Here's how the part is built. I have some questions about the finished solid (model axes, mm). A direction names the side the tool comes from. Round coordinates to 2 decimals unless told otherwise and drop trailing zeros. Write each loop counter-clockwise with the first axis right and the second up, starting at its lowest first coordinate (ties: lowest second). Pieces come first, ordered by that corner, then holes. Notation, with made-up numbers: M 53,1 L 88,1 A19 cw 88,23 Z; hole C -0.5,9.25 d9. An arc over 180 degrees is marked long. Write item = value, one per line. Start each with the question number.
(1) Will these pins go through, and if not, where does the flat tip stop? pin 1 Ø7 at (x, z) = (8, -20) entering from +Y; pin 2 Ø1.6 at (x, z) = (-12.5, -1) entering from -Y; pin 3 Ø3 at (x, y) = (19, 14) entering from -Z; pin 4 Ø8 at (y, z) = (7.5, -13.5) entering from -X.
(2) I want a section at A-A (x = 19.85). List the corners of the cut face in (y, z) for me, and give its area (3 significant figures).
(3) I want a section at C-C (x = 7.05). List the corners of the cut face in (y, z) for me.
(4) I need wall thicknesses on line 1 along X through (y, z) = (21, -1); line 2 along X through (y, z) = (1.05, -41.8); line 3 along Z through (x, y) = (-7.5, 13). Which ranges of each line are inside material? Lowest first, please.
(5) On a 3-axis mill with a long thin cutter (end or side, diameter ignored), from which of +Z, -Z, +X, -X, +Y, -Y can I reach the whole of each face in a straight line? I mean faces 5 (the flat face through (7, 18, -2)), 6 (the flat face through (14.1, 1.6, -19.5)), 7 (the flat face through (32.05, 21, -1)), 8 (the flat face through (-9, 10, -1)), 9 (the cylindrical face through (12.45, 13.45, -0.99)). Say none if no direction works.
(6) I want a section at B-B (y = 21.5). List the corners of the cut face in (x, z) for me, and give its area (3 significant figures).
(7) I want a section at D-D (z = -40.5). List the corners of the cut face in (x, y) for me, and give its area (3 significant figures).
(8) If we mould it in two halves opening along Y, with no side actions, what happens to faces 1 (the flat face through (7, 1, -46)), 2 (the flat face through (7, 11, -1)), 3 (the flat face through (23, 10, -1)), 4 (the flat face through (7, 2, -24))? For each: released by +Y, released by -Y, zero draft, split by the parting line, or undercut.
```python
from build123d import *

# Parameters (mm, degrees)
BASEESB_W      = 14.1
BASEESB_H      = 46
BASE_DEPTH     = 2
FUROSFIXESB_R  = 2.1
FUROSFIX_DEPTH = 2
HOLDER_DEPTH   = 2
FUROSUSESB_R   = 8.55
FUROSUS_DEPTH  = 2


with BuildPart() as part:
    # baseEsb → base (new body)
    with BuildSketch(Plane(origin=(0, 0, 0), x_dir=(1, 0, 0), z_dir=(0, 1, 0))):
        with Locations((7.05, 23)):
            Rectangle(BASEESB_W, BASEESB_H)
    extrude(amount=BASE_DEPTH)

    # furosFixEsb → furosFix (cut)
    with BuildSketch(Plane(origin=(0, 2, 0), x_dir=(1, 0, 0), z_dir=(0, 1, 0))):
        with Locations(Location((7.05, 10.1, 0), (0, 0, 270))):
            Circle(FUROSFIXESB_R)
        with Locations(Location((7.05, 41.8, 0), (0, 0, 270))):
            Circle(FUROSFIXESB_R)
    extrude(amount=-FUROSFIX_DEPTH, mode=Mode.SUBTRACT)

    # holderEsb → holder (add)
    with BuildSketch(Plane.XY):
        Polygon((0, 0), (14.1, 0), (14.1, 10), (32.05, 10), (32.05, 33), (-17.95, 33), (-17.95, 10), (0, 10), align=None)
    extrude(amount=-HOLDER_DEPTH)

    # furosUSesb → furosUS (cut)
    with BuildSketch(Plane.XY):
        with Locations((-5.75, 21.5)):
            Circle(FUROSUSESB_R)
        with Locations(Location((19.85, 21.5, 0), (0, 0, 180))):
            Circle(FUROSUSESB_R)
        with BuildLine():
            Line((4.05, 15.8), (10.05, 15.8))
            ThreePointArc((10.05, 15.8), (12.45, 13.4), (10.05, 11))
            Line((10.05, 11), (4.05, 11))
            ThreePointArc((4.05, 11), (1.65, 13.4), (4.05, 15.8))
        make_face()
    extrude(amount=-FUROSUS_DEPTH, mode=Mode.SUBTRACT)


solid = part.part
```
Returned:
q1.pin_1 = 2
q1.pin_2 = 10
q1.pin_3 = -2
q1.pin_4 = through
q2.outline = M 10,-2 L 12.95,-2 L 12.95,0 L 10,0 Z; M 30.05,-2 L 33,-2 L 33,0 L 30.05,0 Z
q2.area = 11.8 mm²
q3.outline = M 0,-46 L 2,-46 L 2,-43.9 L 0,-43.9 Z; M 0,-39.7 L 2,-39.7 L 2,-12.2 L 0,-12.2 Z; M 0,-8 L 2,-8 L 2,-2 L 11,-2 L 11,0 L 0,0 Z; M 15.8,-2 L 33,-2 L 33,0 L 15.8,0 Z
q4.line_1 = -17.95 to -14.29, 2.79 to 11.31, 28.39 to 32.05
q4.line_2 = 0 to 4.95, 9.15 to 14.1
q4.line_3 = -2 to 0
q5.face_5 = -Z, +X, -X, +Y
q5.face_6 = +Z, -Z, +X, -Y
q5.face_7 = +Z, -Z, +X, +Y, -Y
q5.face_8 = +Z, -Z, -X, -Y
q5.face_9 = +Z, -Z
q6.outline = M -17.95,-2 L -14.3,-2 L -14.3,0 L -17.95,0 Z; M 2.8,-2 L 11.3,-2 L 11.3,0 L 2.8,0 Z; M 28.4,-2 L 32.05,-2 L 32.05,0 L 28.4,0 Z
q6.area = 31.6 mm²
q7.outline = M 0,0 L 5.4,0 L 5.4,2 L 0,2 Z; M 8.7,0 L 14.1,0 L 14.1,2 L 8.7,2 Z
q7.area = 21.6 mm²
q8.face_1 = zero draft
q8.face_2 = undercut
q8.face_3 = released by -Y
q8.face_4 = released by +Y
